Verification items for the finished model (mm, model axes). Give positions to 0.01 mm unless a question says otherwise; leave off trailing zeros. Loops run counter-clockwise (first coordinate to the right, second up) from the corner with the lowest first, then second, coordinate; pieces in that order, holes last. Notation, with made-up numbers: (11.25, 20) - (32.25, 20) arc R19 cw to (32.25, 28) - close; hole circle Ø7 at (-33, 87.5). An arc over 180 degrees is marked (long way). Use one line per item in the form item = value.
```python
from build123d import *

# Parameters (mm, degrees)
SKETCH1_W                      = 190
SKETCH1_H                      = 130
BOSS_EXTRUDE1_DEPTH            = 5
M5_CLEARANCE_HOLE1_D           = 5.8
SKETCH6_R                      = 20
CUT_EXTRUDE1_DEPTH             = 10
F_13_0_13_DIAMETER_SLOT1_DEPTH = 5
CUT_EXTRUDE2_REACH             = 117.217
FILLET1_R                      = 5
M5_CLEARANCE_HOLE2_D           = 5.8


# Read off the part's stored shape, not the designer's step: Ø13.0 (13) Diameter Slot1
with BuildPart() as part:
    # Sketch1 → Boss-Extrude1 (new body)
    with BuildSketch(Plane.XY):
        Rectangle(SKETCH1_W, SKETCH1_H)
    extrude(amount=BOSS_EXTRUDE1_DEPTH)

    # M5 Clearance Hole1 (through all)
    with Locations(Plane.XY.offset(5)):
        with Locations((-40, 6), (40, 6), (-40, -56), (40, -56), (-23.55, 58), (23.55, 58), (-23.55, 10.9), (23.55, 10.9), (-10, -56), (10, -56), (-85, 6), (85, 6), (-85, -56), (85, -56)):
            Hole(M5_CLEARANCE_HOLE1_D / 2)

    # Sketch6 → Cut-Extrude1 (cut)
    with BuildSketch(Plane.XY.offset(5)):
        with Locations((0, 34.5)):
            Circle(SKETCH6_R)
    extrude(amount=-CUT_EXTRUDE1_DEPTH, mode=Mode.SUBTRACT)

    # Ø13.0 (13) Diameter Slot1 outline → Ø13.0 (13) Diameter Slot1 (cut)
    with BuildSketch(Plane.XY):
        with BuildLine():
            ThreePointArc((-52.5, -41.5), (-46, -35), (-52.5, -28.5))
            Line((-52.5, -28.5), (-72.5, -28.5))
            ThreePointArc((-72.5, -28.5), (-79, -35), (-72.5, -41.5))
            Line((-72.5, -41.5), (-52.5, -41.5))
        make_face()
        with BuildLine():
            ThreePointArc((52.5, -28.5), (46, -35), (52.5, -41.5))
            Line((52.5, -41.5), (72.5, -41.5))
            ThreePointArc((72.5, -41.5), (79, -35), (72.5, -28.5))
            Line((72.5, -28.5), (52.5, -28.5))
        make_face()
        with BuildLine():
            ThreePointArc((-52.5, -21.5), (-46, -15), (-52.5, -8.5))
            Line((-52.5, -8.5), (-72.5, -8.5))
            ThreePointArc((-72.5, -8.5), (-79, -15), (-72.5, -21.5))
            Line((-72.5, -21.5), (-52.5, -21.5))
        make_face()
        with BuildLine():
            ThreePointArc((52.5, -8.5), (46, -15), (52.5, -21.5))
            Line((52.5, -21.5), (72.5, -21.5))
            ThreePointArc((72.5, -21.5), (79, -15), (72.5, -8.5))
            Line((72.5, -8.5), (52.5, -8.5))
        make_face()
    extrude(amount=F_13_0_13_DIAMETER_SLOT1_DEPTH, mode=Mode.SUBTRACT)

    # Sketch14 → Cut-Extrude2 (cut, up to next)
    with BuildSketch(Plane(origin=(0, 0, 0), x_dir=(-1, 0, 0), z_dir=(0, 0, -1)), mode=Mode.PRIVATE) as cut_extrude2_sk1:
        Polygon((-40, 65), (-95, 10), (-95, 65), align=None)
    cut_extrude2_tool1 = extrude(cut_extrude2_sk1.sketch, amount=-CUT_EXTRUDE2_REACH, mode=Mode.PRIVATE) & part.part
    # Sketch14 → Cut-Extrude2 (cut, up to next)
    with BuildSketch(Plane(origin=(0, 0, 0), x_dir=(-1, 0, 0), z_dir=(0, 0, -1)), mode=Mode.PRIVATE) as cut_extrude2_sk2:
        Polygon((40, 65), (95, 10), (95, 65), align=None)
    cut_extrude2_tool2 = extrude(cut_extrude2_sk2.sketch, amount=-CUT_EXTRUDE2_REACH, mode=Mode.PRIVATE) & part.part
    add(cut_extrude2_tool1.solids().sort_by_distance((76.666667, 46.666667, 0))[0], mode=Mode.SUBTRACT)
    add(cut_extrude2_tool2.solids().sort_by_distance((-76.666667, 46.666667, 0))[0], mode=Mode.SUBTRACT)

    # Fillet1
    fillet1_edges = [part.edges().sort_by_distance(p)[0] for p in [
        (40, 65, 2.5),
        (95, 10, 2.5),
        (-40, 65, 2.5),
        (-95, 10, 2.5),
        (95, -65, 2.5),
        (-95, -65, 2.5),
    ]]
    fillet(fillet1_edges, radius=FILLET1_R)

    # M5 Clearance Hole2 (through all)
    with Locations(Plane.XY.offset(5)):
        with Locations((62.5, 12.5), (-62.5, 12.5)):
            Hole(M5_CLEARANCE_HOLE2_D / 2)


solid = part.part
```
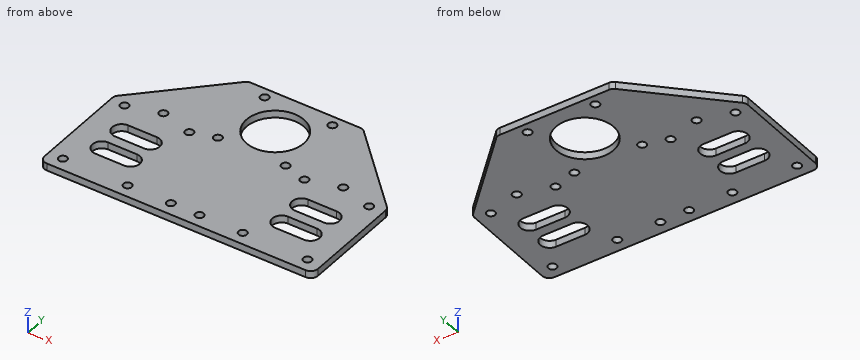
1. Section check B-B, the plane x = -62.5. Record the cut outline in (y, z), then the cut area to 4 significant figures.
Result set:
outline = (-65, 0) - (-41.5, 0) - (-41.5, 5) - (-65, 5) - close; (-28.5, 0) - (-21.5, 0) - (-21.5, 5) - (-28.5, 5) - close; (-8.5, 0) - (9.6, 0) - (9.6, 5) - (-8.5, 5) - close; (15.4, 0) - (42.5, 0) - (42.5, 5) - (15.4, 5) - close
area = 378.5 mm²
2. Scan lines: probe 1 along Y at (x, z) = (85, 2.8); probe 2 along Y at (x, z) = (-65, 1.5); probe 3 along X at (y, z) = (-30.5, 3.4). Record each from-to range of solid material in increasing order.
Result set:
probe_1 = -65 to -58.9, -53.1 to 3.1, 8.9 to 20
probe_2 = -65 to -41.5, -28.5 to -21.5, -8.5 to 11.03, 13.97 to 40
probe_3 = -95 to -77.19, -47.81 to 47.81, 77.19 to 95
3. Section check A-A, the plane x = 23.55. Record the cut outline in (y, z).
Result set:
outline = (-65, 0) - (8, 0) - (8, 5) - (-65, 5) - close; (13.8, 0) - (55.1, 0) - (55.1, 5) - (13.8, 5) - close; (60.9, 0) - (65, 0) - (65, 5) - (60.9, 5) - close
4. Section check C-C, the plane y = 49.5. Record the cut outline in (x, z), then the cut area to 3 significant figures.
Result set:
outline = (-55.5, 0) - (-13.23, 0) - (-13.23, 5) - (-55.5, 5) - close; (13.23, 0) - (55.5, 0) - (55.5, 5) - (13.23, 5) - close
area = 423 mm²
5. Section check D-D, the plane y = -31. Record the cut outline in (x, z), then the cut area to 3 significant figures.
Result set:
outline = (-95, 0) - (-77.62, 0) - (-77.62, 5) - (-95, 5) - close; (-47.38, 0) - (47.38, 0) - (47.38, 5) - (-47.38, 5) - close; (77.62, 0) - (95, 0) - (95, 5) - (77.62, 5) - close
area = 648 mm²
